Can you work these out from the model? Positions are in its coordinate system, mm. Give positions to 0.01 mm unless a question says otherwise; leave off trailing zeros. Loops run counter-clockwise (first coordinate to the right, second up) from the corner with the lowest first, then second, coordinate; pieces in that order, holes last. Notation, with made-up numbers: (20, 65.25) - (77, 65.25) arc R27 cw to (77, 87.25) - close; hole circle Ø9 at (21.25, 49). An arc over 180 degrees is marked (long way). Answer in a Markdown table with one row per item.
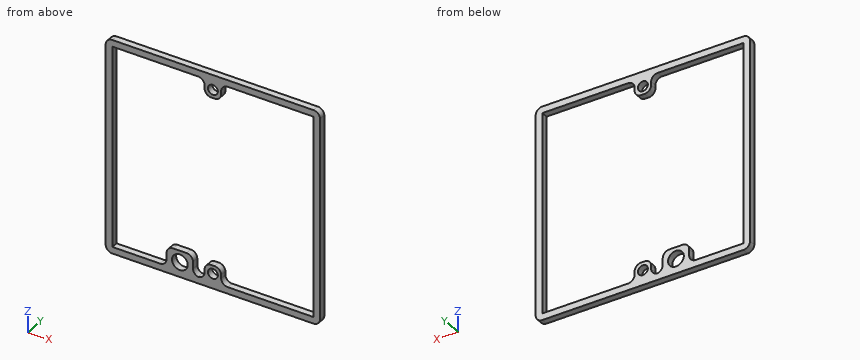
from build123d import *

# Parameters (mm, degrees)
SKETCH1_W           = 64.85
SKETCH1_H           = 64.85
SKETCH1_W_2         = 60.85
SKETCH1_H_2         = 60.85
BOSS_EXTRUDE1_DEPTH = 2
SKETCH2_W           = 5
SKETCH2_H           = 5
SKETCH2_R           = 1.5
BOSS_EXTRUDE2_DEPTH = 2
FILLET1_R           = 2
SKETCH3_W           = 8
SKETCH3_H           = 6
SKETCH3_R           = 2.38125
BOSS_EXTRUDE3_DEPTH = 2
FILLET2_R           = 2


with BuildPart() as part:
    # Sketch1 → Boss-Extrude1 (new body)
    with BuildSketch(Plane(origin=(0, 0, 0), x_dir=(1, 0, 0), z_dir=(0, 1, 0))):
        Rectangle(SKETCH1_W, SKETCH1_H)
        Rectangle(SKETCH1_W_2, SKETCH1_H_2, mode=Mode.SUBTRACT)
    extrude(amount=BOSS_EXTRUDE1_DEPTH)

    # Sketch2 → Boss-Extrude2 (add)
    # profile 1 of 2: a face of its own
    with BuildSketch(Plane(origin=(0, 2, 0), x_dir=(1, 0, 0), z_dir=(0, 1, 0))):
        with Locations((0, 27.925)):
            Rectangle(SKETCH2_W, SKETCH2_H)
        with Locations(Location((0, 27.925, 0), (0, 0, 270))):
            Circle(SKETCH2_R, mode=Mode.SUBTRACT)
    # profile 2 of 2: a face of its own
    with BuildSketch(Plane(origin=(0, 2, 0), x_dir=(1, 0, 0), z_dir=(0, 1, 0))):
        with Locations((0, -27.925)):
            Rectangle(SKETCH2_W, SKETCH2_H)
        with Locations(Location((0, -27.925, 0), (0, 0, 270))):
            Circle(SKETCH2_R, mode=Mode.SUBTRACT)
    extrude(amount=-BOSS_EXTRUDE2_DEPTH)

    # Fillet1
    fillet1_edges = [part.edges().sort_by_distance(p)[0] for p in [
        (32.425, 1, 32.425),
        (-32.425, 1, 32.425),
        (32.425, 1, -32.425),
        (-32.425, 1, -32.425),
        (2.5, 1, -30.425),
        (-2.5, 1, -30.425),
        (-2.5, 1, 30.425),
        (2.5, 1, 30.425),
        (2.5, 1, -25.425),
        (-2.5, 1, -25.425),
        (-2.5, 1, 25.425),
        (2.5, 1, 25.425),
    ]]
    fillet(fillet1_edges, radius=FILLET1_R)

    # Sketch3 → Boss-Extrude3 (add)
    with BuildSketch(Plane(origin=(0, 2, 0), x_dir=(1, 0, 0), z_dir=(0, 1, 0))):
        with Locations((-10, 27.425)):
            Rectangle(SKETCH3_W, SKETCH3_H)
        with Locations(Location((-10, 27.925, 0), (0, 0, 270))):
            Circle(SKETCH3_R, mode=Mode.SUBTRACT)
    extrude(amount=-BOSS_EXTRUDE3_DEPTH)

    # Fillet2
    # the kernel refuses this fillet: 2 mm, written as the material it adds along each edge
    with BuildSketch(Plane(origin=(-14, 2, -30.425), x_dir=(-1, 0, 0), z_dir=(0, -1, 0))) as fillet2_piece_1:
        with BuildLine():
            CenterArc((FILLET2_R, -FILLET2_R), FILLET2_R, 90, 90)
            Line((0, -FILLET2_R), (0, 0))
            Line((0, 0), (FILLET2_R, 0))
        make_face()
    extrude(amount=2)
    with BuildSketch(Plane(origin=(-6, 2, -30.425), x_dir=(1, 0, 0), z_dir=(0, -1, 0))) as fillet2_piece_2:
        with BuildLine():
            CenterArc((2, 1.936491673), FILLET2_R, 180, 75.522487814)
            Line((0, 1.936491673), (0, 0))
            Line((0, 0), (1.5, 0))
        make_face()
    extrude(amount=2)
    # the kernel refuses this fillet: 2 mm, written as the material it takes off along each edge
    with BuildSketch(Plane(origin=(-14, 7, -24.425), x_dir=(1, 0, 0), z_dir=(0, -1, 0)), Plane(origin=(-6, 7, -24.425), x_dir=(0, 0, -1), z_dir=(0, -1, 0))) as fillet2_2_piece_1:
        with BuildLine():
            CenterArc((FILLET2_R, -FILLET2_R), FILLET2_R, 90, 90)
            Line((0, -FILLET2_R), (0, 0))
            Line((0, 0), (FILLET2_R, 0))
        make_face()
    extrude(amount=12, mode=Mode.SUBTRACT)


solid = part.part
Q1. Imagine slicing it at B-B, the plane z = -22.5. Write out the boundary of the cut face in (x, y) (3 decimals).
Checked values:
| item | result |
|---|---|
| outline | (-32.425, 0) - (-30.425, 0) - (-30.425, 2) - (-32.425, 2) - close; (30.425, 0) - (32.425, 0) - (32.425, 2) - (30.425, 2) - close |
Q2. Imagine slicing it at C-C, the plane x = -9. Write out the boundary of the cut face in (y, z) (3 decimals).
Checked values:
| item | result |
|---|---|
| outline | (0, -32.425) - (2, -32.425) - (2, -30.086) - (0, -30.086) - close; (0, -25.764) - (2, -25.764) - (2, -24.425) - (0, -24.425) - close; (0, 30.425) - (2, 30.425) - (2, 32.425) - (0, 32.425) - close |
Q3. If I drill on line 1 (X direction, y = 0.2, z = 17) (3 decimals); line 2 (X direction, y = 1.7, z = -30) (3 decimals), over which ranges is the centre line in solid material (lowest first)? Write a range as [from, to].
Checked values:
| item | result |
|---|---|
| line 1 | x = [-32.425, -30.425], [30.425, 32.425] |
| line 2 | x = [-32.425, -30.425], [-14.767, -11.168], [-8.832, -5.31], [-3.267, 3.267], [30.425, 32.425] |
Q4. Imagine slicing it at A-A, the plane x = -17. Write out the boundary of the cut face in (y, z) (3 decimals).
Checked values:
| item | result |
|---|---|
| outline | (0, -32.425) - (2, -32.425) - (2, -30.425) - (0, -30.425) - close; (0, 30.425) - (2, 30.425) - (2, 32.425) - (0, 32.425) - close |
Q5. For pin 1 (5.5 mm diameter, centred on x = -10, z = -27.925, fed in from -Y), with a flat end and sliding along its axis, tell me the tip position at first contact or that it passes through.
Checked values:
| item | result |
|---|---|
| pin 1 | stops at y = 0 |
Q6. Imagine slicing it at D-D, the plane y = 1.25. Count the separate pieces of the cut face and the enclosed holes in it, and give its area (3 significant figures).
Checked values:
| item | result |
|---|---|
| separate pieces | 1 |
| enclosed holes | 4 |
| area | 565 mm² |
